Source: CAD feature listing. Evaluate the final solid. Frame: model axes, mm. Give positions to 0.01 mm unless a question says otherwise; leave off trailing zeros. Loops run counter-clockwise (first coordinate to the right, second up) from the corner with the lowest first, then second, coordinate; pieces in that order, holes last.
```python
from build123d import *

# Parameters (mm, degrees)
SKETCH1_R           = 2.5
SKETCH1_W           = 40
SKETCH1_H           = 50
SKETCH1_H_2         = 60
BOSS_EXTRUDE1_DEPTH = 4


with BuildPart() as part:
    # Sketch1 → Boss-Extrude1 (new body)
    with BuildSketch(Plane(origin=(0, 0, 0), x_dir=(1, 0, 0), z_dir=(0, 1, 0))):
        Polygon((-48, 102.368421053), (-48, 0), (50, 0), (50, 100), (130, 77.738349066), (130, -100), (-128, -100), (-128, 75), align=None)
        with Locations(Location((-114, -90, 0), (0, 0, 270))):
            Circle(SKETCH1_R, mode=Mode.SUBTRACT)
        with Locations(Location((-68, -86, 0), (0, 0, 270))):
            Circle(SKETCH1_R, mode=Mode.SUBTRACT)
        with Locations(Location((-18, -86, 0), (0, 0, 270))):
            Circle(SKETCH1_R, mode=Mode.SUBTRACT)
        with Locations(Location((-120, 62, 0), (0, 0, 270))):
            Circle(SKETCH1_R, mode=Mode.SUBTRACT)
        with Locations(Location((-114, -23, 0), (0, 0, 270))):
            Circle(SKETCH1_R, mode=Mode.SUBTRACT)
        with Locations(Location((18, -86, 0), (0, 0, 90))):
            Circle(SKETCH1_R, mode=Mode.SUBTRACT)
        with Locations(Location((68, -86, 0), (0, 0, 90))):
            Circle(SKETCH1_R, mode=Mode.SUBTRACT)
        with Locations(Location((114, -90, 0), (0, 0, 90))):
            Circle(SKETCH1_R, mode=Mode.SUBTRACT)
        with Locations(Location((114, -23, 0), (0, 0, 90))):
            Circle(SKETCH1_R, mode=Mode.SUBTRACT)
        with Locations(Location((120, 62, 0), (0, 0, 90))):
            Circle(SKETCH1_R, mode=Mode.SUBTRACT)
        with Locations((95, -60)):
            Rectangle(SKETCH1_W, SKETCH1_H, mode=Mode.SUBTRACT)
        with Locations((95, 40)):
            Rectangle(SKETCH1_W, SKETCH1_H_2, mode=Mode.SUBTRACT)
        with Locations((-96, 40)):
            Rectangle(SKETCH1_W, SKETCH1_H_2, mode=Mode.SUBTRACT)
        with Locations((-93, -60)):
            Rectangle(SKETCH1_W, SKETCH1_H, mode=Mode.SUBTRACT)
    extrude(amount=BOSS_EXTRUDE1_DEPTH)


solid = part.part
```
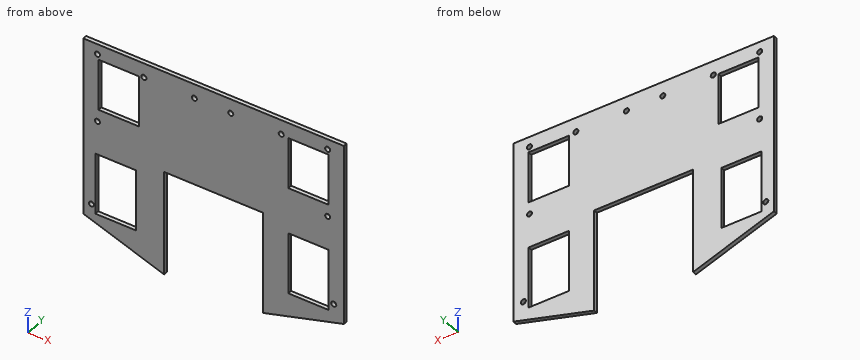
(1) Section A-A, the plane z = 73. Return the cut outline in (x, y), then the cut area to 3 significant figures.
A:
outline: (-128, 0) - (-113, 0) - (-113, 4) - (-128, 4) - close; (-73, 0) - (75, 0) - (75, 4) - (-73, 4) - close; (115, 0) - (130, 0) - (130, 4) - (115, 4) - close
area: 712 mm2
(2) Section C-C, the plane z = -27.5. Return the cut outline in (x, y), then the cut area to 3 significant figures.
A:
outline: (-128, 0) - (-116, 0) - (-116, 4) - (-128, 4) - close; (-76, 0) - (-48, 0) - (-48, 4) - (-76, 4) - close; (50, 0) - (75, 0) - (75, 4) - (50, 4) - close; (115, 0) - (130, 0) - (130, 4) - (115, 4) - close
area: 320 mm2
(3) Section B-B, the plane y = 0.7. Count the separate pieces of the cut face and the enclosed holes in it, then the cut area to 3 significant figures.
A:
separate pieces: 1
enclosed holes: 14
area: 31,000 mm2
(4) First-contact query: pin 1 (2 mm diameter, centred on x = 96.5, y = 2.5, fed in from -Z); pin 2 (2 mm diameter, centred on x = -99.5, y = 2, fed in from -Z). Flat tips, straight axial feed; report the tip coordinate or a pass-through.
A:
pin 1: stops at z = -87.34
pin 2: stops at z = -85.09
(5) Ray query, line 1 along X through (y, z) = (3.85, 51.5); line 2 along X through (y, z) = (3, 90); line 3 along X through (y, z) = (0.3, -39). Return the intervals inside material, ascending.
A:
line 1: x = -128 to -113, -73 to 75, 115 to 130
line 2: x = -128 to -116.5, -111.5 to 111.5, 116.5 to 130
line 3: x = -128 to -116, -76 to -48, 50 to 75, 115 to 130
